Autodesk Inventor part; units mm, degrees
ref_plane "SC_XY" through (0, 0, 0) normal (0, 0, 1) x (-1, 0, 0)
ref_plane "SC_YZ" through (0, 0, 0) normal (-1, 0, 0) x (0, -1, 0)
ref_plane "SC_ZX" through (0, 0, 0) normal (0, -1, 0) x (0, 0, 1)
sketch "Sketch_12" plane through (0, 0, 0) normal (0, 1, 0) x (-1, 0, 0)
  line L0 (5.5, 3.4) -> (-1.2, 3.4)
  line L1 (-1.2, 3.4) -> (-6, 5.984)
  line L2 (-6, 5.984) -> (-6, 1.5)
  line L3 (-6, 1.5) -> (5.5, 1.5)
  line L4 (5.5, 1.5) -> (5.5, 3.4)
extrude "Extrusion1" add sketch "Sketch_12" along normal mid plane 17.3
sketch "Sketch_16" plane through (0, 0, 0) normal (0, 0, 1) x (1, 0, 0)
  circle A0 centre (0, 0) radius 3.5
extrude "Extrusion2" cut sketch "Sketch_16" along normal blind 6
sketch "Sketch_1" plane through (0, 0, 0) normal (0, 1, 0) x (0, 0, 1)
  line L0 (0, 7.5) -> (0, -7)
  line L1 (0, -7) -> (4, -7)
  line L2 (4, -7) -> (4, -5.5)
  line L3 (4, -5.5) -> (1.5, -5.5)
  line L4 (1.5, -5.5) -> (1.5, 6)
  line L5 (1.5, 6) -> (7.1676, 6)
  line L6 (7.1676, 6) -> (10.6991, 7.3911)
  arc A0 (9.0682, 5.2618) -> (10.6991, 7.3911) centre (11.652, 4.972) ccw
  line L7 (9.0682, 5.2618) -> (7.5776, 5.429)
  arc A1 (7.5776, 5.429) -> (10.1493, 8.7867) centre (11.652, 4.972) ccw
  line L8 (10.1493, 8.7867) -> (6.8828, 7.5)
  line L9 (6.8828, 7.5) -> (0, 7.5)
extrude "Extrusion3" add sketch "Sketch_1" along normal mid plane 60
sketch "Sketch_8" plane through (0, 22.5, 0) normal (0, 1, 0) x (0, 0, 1)
  arc A0 (7.1855, 5.5204) -> (8.6409, 1.6278) centre (11.652, 4.972) ccw
  line L0 (8.6409, 1.6278) -> (9.9792, 3.1141)
  arc A1 (9.9792, 3.1141) -> (13.622, 6.5112) centre (11.652, 4.972) ccw
  line L1 (13.622, 6.5112) -> (15.198, 7.7425)
  arc A2 (15.198, 7.7425) -> (10.2614, 9.2518) centre (11.652, 4.972) ccw
  line L2 (10.2614, 9.2518) -> (10.8795, 7.3496)
  arc A3 (10.8795, 7.3496) -> (9.1706, 5.2767) centre (11.652, 4.972) ccw
  line L3 (9.1706, 5.2767) -> (7.1855, 5.5204)
extrude "Extrusion4" cut sketch "Sketch_8" along normal mid plane 5
sketch "Sketch_9" plane through (0, -22.5, 0) normal (0, 1, 0) x (0, 0, 1)
  arc A0 (7.1855, 5.5204) -> (8.6409, 1.6278) centre (11.652, 4.972) ccw
  line L0 (8.6409, 1.6278) -> (9.9792, 3.1141)
  arc A1 (9.9792, 3.1141) -> (13.622, 6.5112) centre (11.652, 4.972) ccw
  line L1 (13.622, 6.5112) -> (15.198, 7.7425)
  arc A2 (15.198, 7.7425) -> (10.2614, 9.2518) centre (11.652, 4.972) ccw
  line L2 (10.2614, 9.2518) -> (10.8795, 7.3496)
  arc A3 (10.8795, 7.3496) -> (9.1706, 5.2767) centre (11.652, 4.972) ccw
  line L3 (9.1706, 5.2767) -> (7.1855, 5.5204)
extrude "Extrusion5" cut sketch "Sketch_9" along normal mid plane 5
sketch "Sketch_5" plane through (0, 0, 0) normal (0, 1, 0) x (0, 0, 1)
  line L0 (1.5, 0) -> (0, 0)
  line L1 (0, 0) -> (0, 2.517)
  arc A0 (0, 2.517) -> (0.45, 2.067) centre (0.45, 2.517) ccw
  line L2 (0.45, 2.067) -> (1.5, 2.067)
  line L3 (1.5, 2.067) -> (1.5, 0)
  line L4 (1.5, 0) -> (0, 0)
revolve "Revolution1" cut sketch "Sketch_5" angle 360 about axis through (0, 0, 1.5) along (0, 0, 1)
thread "Thread1"
sketch "Sketch_6" plane through (7.5, 0, 0) normal (-1, 0, 0) x (0, 0, 1)
  line L0 (5.984, -10.5) -> (15.984, -10.5)
  line L1 (15.984, -10.5) -> (15.984, 10.5)
  line L2 (15.984, 10.5) -> (5.984, 10.5)
  line L3 (5.984, 10.5) -> (5.984, -10.5)
extrude "Extrusion6" cut sketch "Sketch_6" along normal mid plane 14
sketch "Sketch_7" plane through (0, 0, 11.652) normal (0, 0, 1) x (1, 0, 0)
  line L0 (4.972, -32.2) -> (4.972, 33.8)
  line L1 (4.972, 33.8) -> (6.472, 33.8)
  line L2 (6.472, 33.8) -> (7.472, 31.05)
  line L3 (7.472, 31.05) -> (7.472, -26.7)
  line L4 (7.472, -26.7) -> (7.572, -26.7)
  line L5 (7.572, -26.7) -> (7.572, -27.7)
  line L6 (7.572, -27.7) -> (6.722, -27.7)
  line L7 (6.722, -27.7) -> (6.722, -30.7)
  line L8 (6.722, -30.7) -> (7.972, -30.7)
  line L9 (7.972, -30.7) -> (7.972, -32.2)
  line L10 (7.972, -32.2) -> (4.972, -32.2)
  line L11 (4.972, -32.2) -> (4.972, 33.8)
revolve "Revolution2" add sketch "Sketch_7" angle 360 about axis through (4.972, -32.2, 11.652) along (0, -1, 0)
ref_plane "SC_XY" through (0, 0, 0) normal (0, 0, 1) x (-1, 0, 0)
ref_plane "SC_YZ" through (0, 0, 0) normal (-1, 0, 0) x (0, -1, 0)
ref_plane "SC_ZX" through (0, 0, 0) normal (0, -1, 0) x (0, 0, 1)
ref_plane "TUER1_XY" through (4.972, 0, 11.652) normal (0, -1, 0) x (0, 0, 1)
ref_plane "TUER1_YZ" through (4.972, 0, 11.652) normal (0, 0, 1) x (-1, 0, 0)
ref_plane "TUER1_ZX" through (4.972, 0, 11.652) normal (-1, 0, 0) x (0, -1, 0)
ref_plane "TUER2_XY" through (4.972, 0, 11.652) normal (0, 1, 0) x (0, 0, 1)
ref_plane "TUER2_YZ" through (4.972, 0, 11.652) normal (0, 0, 1) x (1, 0, 0)
ref_plane "TUER2_ZX" through (4.972, 0, 11.652) normal (1, 0, 0) x (0, 1, 0)
properties part number "1XXX_01_04(T,2)_P7"
For this review, take the finished solid that the model builds, in its own axes (mm). A direction names the side the tool comes from. Give positions to 0.01 mm unless a question says otherwise; leave off trailing zeros. Loops run counter-clockwise (first coordinate to the right, second up) from the corner with the lowest first, then second, coordinate; pieces in that order, holes last. Notation, with made-up numbers: M 21,86.5 L 77,86.5 A25 cw 77,98.5 Z; hole C 62.5,-9.5 d1. An arc over 180 degrees is marked long. Put each result on its own line as item: value. Start each with the question number.
(1) Add section C-C, the plane y = 0. Write out the cut boundary in (x, z), then the cut area to 3 significant figures.
(2) The part is to be moulded in two halves that separate along Z. For faces 6 (the cylindrical face through (7.74, -31.46, 10.5)), 7 (the flat face through (5, 33.8, 12)), 8 (the flat face through (2, -8.65, 3)), say which applies: +Z half, -Z half, draft (parallel to the pull), parting line (faces both ways), or undercut.
(3) Wall thickness on L1, parallel to Y at x = 3, z = 9; L2, parallel to X at y = 0, z = 3.45; L3, parallel to Y at x = 0, z = 3: over which ranges is each line inside the solid? List them lowest first.
(4) For pin 1 (2 mm diameter, centred on x = -1.5, z = 4, fed in from -Y); pin 2 (2 mm diameter, centred on x = 6.5, y = 6.5, fed in from +Z); pin 3 (5 mm diameter, centred on x = -1.5, z = 3.5, fed in from +Y), all flat-tipped, find the tip position at first contact; note any pin that passes through.
(5) Machinability: for faces 1 (the flat face through (2.47, -22.54, 9.4)), 2 (the flat face through (7.028, -22.535, 14.284)), 3 (the flat face through (6, -19, 4)), 4 (the flat face through (5.344, -15.317, 8.333)), 5 (the flat face through (-5.5, -0.4, 3.6)), which of the approach directions +Z, -Z, +X, -X, +Y, -Y give a long, thin tool a straight path to every point of the face, cutting with its end or side? Answer none if there is none.
(6) Add section B-B, the plane y = -21. Write out the cut boundary in (x, z), then the cut area to 3 significant figures.
(7) Add section A-A, the plane x = 0. Write out the cut boundary in (y, z).
Result:
1. outline: M -7,0 L -2.52,0 A0.45 ccw -2.07,0.45 L -2.07,1.5 L -3.5,1.5 L -3.5,3.4 L -5.5,3.4 L -5.5,4 L -7,4 Z; M 2.07,0.45 A0.45 ccw 2.52,0 L 7.5,0 L 7.5,5.98 L 6,5.98 L 3.5,4.64 L 3.5,1.5 L 2.07,1.5 Z; C 4.97,11.65 d5
1. area: 58.9 mm^2
2. face 6: parting line
2. face 7: draft
2. face 8: undercut
3. L1: y = -30 to -25, -20 to -10.5, 10.5 to 20, 25 to 30
3. L2: x = -7 to -5.5, 3.5 to 7.5
3. L3: y = -8.65 to -3.5, 3.5 to 8.65
4. pin 1: stops at y = -8.65
4. pin 2: stops at z = 14.1
4. pin 3: stops at y = 30
5. face 1: none
5. face 2: +X
5. face 3: -Y
5. face 4: +Y
5. face 5: +Z
6. outline: M -7,0 L 7.5,0 L 7.5,6.88 L 8.79,10.15 A4.1 ccw 8.87,10.39 L 7.44,10.85 A2.6 cw 7.39,10.7 L 6,7.17 L 6,1.5 L -5.5,1.5 L -5.5,4 L -7,4 Z; M 1.93,8.91 L 3.04,9.91 A2.6 cw 6.57,13.7 L 7.5,14.88 A4.1 ccw Z; C 4.97,11.65 d5
6. area: 74.1 mm^2
7. outline: M -30,0 L -2.52,0 A0.45 ccw -2.07,0.45 L -2.07,1.5 L -3.5,1.5 L -3.5,3.4 L -8.65,3.4 L -8.65,1.5 L -30,1.5 Z; M 2.07,0.45 A0.45 ccw 2.52,0 L 30,0 L 30,1.5 L 8.65,1.5 L 8.65,3.4 L 3.5,3.4 L 3.5,1.5 L 2.07,1.5 Z
